The model under review builds one solid part; all positions refer to its coordinate system, in mm. Give positions to 0.01 mm unless a question says otherwise; leave off trailing zeros. Order: outer loops, then holes, each group sorted by start corner. A loop starts at its lowest first (then second) coordinate and runs counter-clockwise, first axis right, second up.
Autodesk Fusion 360 part; units mm, degrees
sketch "Sketch1" plane through (0, 0, 0) normal (0, 1, 0) x (1, 0, 0)
  line L0 (5, 27.5) -> (-5, 27.5)
  line L1 (-5, 27.5) -> (-5, -27.5)
  line L2 (-5, -27.5) -> (5, -27.5)
  line L3 (5, -27.5) -> (5, 27.5)
  line L4 (5, 27.5) -> (-5, -27.5) construction
  line L5 (-5, 27.5) -> (5, -27.5) construction
  line L6 (0, -24.05) -> (0, -22.5)
  circle A0 centre (0, -22.5) radius 1.55
  circle A1 centre (0, 22.5) radius 1.55
  dimension "d1" = 10
  dimension "d2" = 55
  dimension "d4" = 3.1
extrude "Extrude1" add sketch "Sketch1" along normal blind 5
sketch "Sketch2" plane through (0, 0, -27.5) normal (0, 0, -1) x (1, 0, 0)
  line L0 (5, 0) -> (-5, 0)
  line L1 (-5, 0) -> (-5, -5)
  line L2 (-5, -5) -> (5, -5)
  line L3 (5, -5) -> (5, 0)
  circle A0 centre (0, -2.5) radius 1.75
  dimension "d7" = 2.5
  dimension "d8" = 3.5
extrude "Extrude2" cut sketch "Sketch2" against normal blind 2 contours A0
extrude "Extrude3" add 1 faces at (3.9167, 2.5, -27.5) along direction (0, 0, -1) blind 6
extrude "Extrude4" add 1 faces at (-0.3896, 1.8511, -25.5) along direction (0, 0, -1) blind 2
extrude "Extrude5" add 1 faces at (-0.0386, 5, -30.3486) along direction (0, 1, 0) blind 1
extrude "Extrude6" add 1 faces at (-0.0386, 0, -30.3486) along direction (0, -1, 0) blind 1
Item 1: For line 1 (Z direction, x = 0, y = 1); line 2 (X direction, y = 2.5, z = -22.5); line 3 (Y direction, x = 0, z = -31.6), list the stretches that pass through material, from the lowest coordinate up.
Values found:
line 1: z = -27.5 to -24.05, -20.95 to 20.95, 24.05 to 27.5
line 2: x = -5 to -1.55, 1.55 to 5
line 3: y = -1 to 0.75, 4.25 to 6
Item 2: Take a section at B-B (y = 1.75). Give the boundary of the cut face in (x, z).
Values found:
outline: (-5, -33.5) - (-1.58, -33.5) - (-1.58, -27.5) - (1.58, -27.5) - (1.58, -33.5) - (5, -33.5) - (5, 27.5) - (-5, 27.5) - close; hole circle Ø3.1 at (0, -22.5); hole circle Ø3.1 at (0, 22.5)
Item 3: Take a section at C-C (x = -1). Give the boundary of the cut face in (y, z).
Values found:
outline: (-1, -33.5) - (1.06, -33.5) - (1.06, -27.5) - (3.94, -27.5) - (3.94, -33.5) - (6, -33.5) - (6, -23.68) - (-1, -23.68) - close; (-1, -21.32) - (6, -21.32) - (6, 21.32) - (-1, 21.32) - close; (-1, 23.68) - (6, 23.68) - (6, 27.5) - (-1, 27.5) - close
Item 4: Draft analysis for pull direction Y (two halves, no side actions). For faces 1 (the cylindrical face through (0.81, 0.95, -30.46)), 2 (the cylindrical face through (-0.202, 2.549, -24.037)), 3 (the flat face through (0, -1, -3)), 4 (the flat face through (0, 2, -27.5)), state which applies: released by +Y, released by -Y, zero draft, split by the parting line, or undercut.
Values found:
face 1: undercut
face 2: zero draft
face 3: released by -Y
face 4: undercut
Item 5: Take a section at A-A (z = -22.5). Give the boundary of the cut face in (x, y), and give its area (3 significant figures).
Values found:
outline: (-5, -1) - (-1.55, -1) - (-1.55, 6) - (-5, 6) - close; (1.55, -1) - (5, -1) - (5, 6) - (1.55, 6) - close
area: 48.3 mm2
Item 6: Clearance check with a flat-ended pin moving along its axis: pin 1 Ø1 at (x, y) = (-0.5, 3.5) entering from -Z. State where the tip first meets the part, or that it passes through.
Values found:
pin 1: stops at z = -27.5
